from build123d import *

# Parameters (mm, degrees)
F0_W     = 152.4
F0_H     = 50.8
F1_DEPTH = 76.2
F3_DEPTH = 76.2
F5_DEPTH = 76.2
F7_DEPTH = 152.4


with BuildPart() as f1:
    # F0 (on Front) → F1 (new body)
    with BuildSketch(Plane.XZ):
        with Locations((76.2, -25.4)):
            Rectangle(F0_W, F0_H)
    extrude(amount=F1_DEPTH)

    # F2 (on face) → F3 (cut)
    with BuildSketch(Plane.XZ.offset(76.2)):
        Polygon((152.4, -12.7), (152.4, 0), (88.9, 0), (101.6, -12.7), align=None)
    extrude(amount=-F3_DEPTH, mode=Mode.SUBTRACT)

    # F4 (on face) → F5 (cut)
    with BuildSketch(Plane.XZ.offset(76.2)):
        Polygon((63.5, 0), (25.4, 0), (25.4, -12.7), (12.7, -12.7), (12.7, -25.4), (76.2, -25.4), (76.2, -12.7), (63.5, -12.7), align=None)
    extrude(amount=-F5_DEPTH, mode=Mode.SUBTRACT)

    # F6 (on face) → F7 (cut)
    with BuildSketch(Plane.YZ.offset(152.4)):
        Polygon((-63.497171, -38.1), (-50.8, -50.8), (-25.4, -50.8), (-12.691214, -38.1), (-25.4, -38.1), (-50.8, -38.1), align=None)
    extrude(amount=-F7_DEPTH, mode=Mode.SUBTRACT)


solid = f1.part
CAD build for the part. Positions are in the model's coordinates, mm. A direction names the side the tool comes from. Round coordinates to 2 decimals unless told otherwise and drop trailing zeros. Write each loop counter-clockwise with the first axis right and the second up, starting at its lowest first coordinate (ties: lowest second). Pieces come first, ordered by that corner, then holes. Notation, with made-up numbers: M -33.75,1 L 9.25,1 A15 ccw 9.25,30 Z; hole C 56,89.25 d8. An arc over 180 degrees is marked long. Put each result on its own line as item: value. Start each with the question number.
1) Drill centre lines: probe 1 along Z at (x, y) = (73, -46.5); probe 2 along X at (y, z) = (-28, -20); probe 3 along Z at (x, y) = (44.5, -70.5). Where is each one in solid material? Low to high. Write a range as [from, to].
2) Pin check, flat tips, straight feed: pin 1 Ø12 at (x, z) = (105.5, -7.5) entering from +Y; pin 2 Ø6.5 at (y, z) = (-36, -7) entering from +X; pin 3 Ø2 at (x, y) = (45.5, -26) entering from +Z; pin 4 Ø4 at (x, y) = (86, -32.5) entering from -Z. Stop position of each tip, or through.
3) Saw through at A-A, the plane z = -21. Write the cut outline in (x, y), and give its area (3 significant figures).
4) Saw through at D-D, the plane y = -20.5. Write the cut outline in (x, z), and give its area (3 significant figures).
5) Saw through at C-C, the plane x = 80. Write the cut outline in (y, z), and give its area (3 significant figures).
6) Pull direction Z, two halves, no side cores. Call faces 4 (the flat face through (76.2, -39, -19)), 5 (the flat face through (25.4, -39, -6)), 6 (the flat face through (95.2, -38.6, -6.3)): pulls with the +Z half, pulls with the -Z half, needs draft (parallel to the pull), parting line crosses it, or undercut.
7) 3-axis set-ups, long thin cutter, end or side, ignore diameter. For faces 1 (the flat face through (12.7, -39, -19)), 2 (the flat face through (63.5, -39, -6)), 3 (the flat face through (77, -38, -38.1)): which of +Z, -Z, +X, -X, +Y, -Y reach the whole face in a straight line?
8) Saw through at B-B, the plane y = -8.5. Write the cut outline in (x, z), and give its area (3 significant figures).
Resolved:
1. probe 1: [-38.1, -25.4], [-12.7, 0]
1. probe 2: [0, 12.7], [76.2, 152.4]
1. probe 3: [-50.8, -25.4]
2. pin 1: y = 0
2. pin 2: x = 99.15
2. pin 3: z = -25.4
2. pin 4: z = -38.1
3. outline: M 0,-76.2 L 12.7,-76.2 L 12.7,0 L 0,0 Z; M 76.2,-76.2 L 152.4,-76.2 L 152.4,0 L 76.2,0 Z
3. area: 6,770 mm²
4. outline: M 0,-50.8 L 152.4,-50.8 L 152.4,-45.9 L 0,-45.9 Z; M 0,-38.1 L 152.4,-38.1 L 152.4,-12.7 L 101.6,-12.7 L 88.9,0 L 63.5,0 L 63.5,-12.7 L 76.2,-12.7 L 76.2,-25.4 L 12.7,-25.4 L 12.7,-12.7 L 25.4,-12.7 L 25.4,0 L 0,0 Z
4. area: 4,540 mm²
5. outline: M -76.2,-50.8 L -50.8,-50.8 L -63.5,-38.1 L -12.69,-38.1 L -25.4,-50.8 L 0,-50.8 L 0,0 L -76.2,0 Z
5. area: 3,390 mm²
6. face 4: undercut
6. face 5: needs draft
6. face 6: pulls with the +Z half
7. face 1: +Y, -Y
7. face 2: +Z, +Y, -Y
7. face 3: +X, -X
8. outline: M 0,-50.8 L 152.4,-50.8 L 152.4,-12.7 L 101.6,-12.7 L 88.9,0 L 63.5,0 L 63.5,-12.7 L 76.2,-12.7 L 76.2,-25.4 L 12.7,-25.4 L 12.7,-12.7 L 25.4,-12.7 L 25.4,0 L 0,0 Z
8. area: 5,730 mm²
